```python
from build123d import *

# Parameters (mm, degrees)
SKETCH021_R     = 3.65
SKETCH021_R_2   = 1.6
SKETCH021_W     = 6.5
SKETCH021_H     = 3
SKETCH021_W_2   = 11.5
PAD009_DEPTH    = 9.5
POCKET012_DEPTH = 7
POCKET010_DEPTH = 3.5
SKETCH022_W     = 25.7
SKETCH022_H     = 13
POCKET011_DEPTH = 3
SKETCH023_R     = 1.8
POCKET009_DEPTH = 1.5
FILLET006_R     = 1
FILLET007_R     = 0.99
FILLET008_R     = 0.5


with BuildPart() as part:
    # Sketch021 → Pad009 (new body)
    with BuildSketch(Plane.XY):
        with BuildLine():
            Line((15.5, -31.35), (15.5, -7.25))
            Line((15.5, -7.25), (11, -7.25))
            Line((11, -7.25), (11, 7.25))
            Line((11, 7.25), (15.5, 7.25))
            Line((15.5, 7.25), (15.5, 11.85))
            Line((15.5, 11.85), (-5.5, 11.85))
            ThreePointArc((-5.5, 11.85), (-12.571068, 8.921068), (-15.5, 1.85))
            Line((-15.5, 1.85), (-15.5, -25.57))
            ThreePointArc((-15.5, -25.57), (-14.679899, -27.549899), (-12.7, -28.37))
            Line((-9.7, -28.37), (-12.7, -28.37))
            Line((-9.7, -29.49), (-9.7, -28.37))
            Line((-9.7, -29.49), (7, -29.49))
            Line((7, -29.49), (7, -31.35))
            Line((7, -31.35), (15.5, -31.35))
        make_face()
        Circle(SKETCH021_R, mode=Mode.SUBTRACT)
        with Locations((-11, -12.5)):
            Circle(SKETCH021_R_2, mode=Mode.SUBTRACT)
        with Locations((11, -12.5)):
            Circle(SKETCH021_R_2, mode=Mode.SUBTRACT)
        with Locations((-6, 8.5)):
            Circle(SKETCH021_R_2, mode=Mode.SUBTRACT)
        with Locations((8, 8.5)):
            Circle(SKETCH021_R_2, mode=Mode.SUBTRACT)
        with Locations((-8.91, -25.81)):
            Rectangle(SKETCH021_W, SKETCH021_H, mode=Mode.SUBTRACT)
        with Locations((6.35, -25.81)):
            Rectangle(SKETCH021_W_2, SKETCH021_H, mode=Mode.SUBTRACT)
    extrude(amount=PAD009_DEPTH)

    # Sketch019 (on Face29 of Pad009) → Pocket012 (cut)
    with BuildSketch(Plane.XY.offset(9.5)):
        Polygon((8.25, -4), (6.25, -4), (6.25, -6.25), (-6.25, -6.25), (-6.25, -4), (-8.25, -4), (-8.25, 4), (-6.25, 4), (-6.25, 6.25), (6.25, 6.25), (6.25, 4), (8.25, 4), align=None)
    extrude(amount=-POCKET012_DEPTH, mode=Mode.SUBTRACT)

    # Sketch020 (on Face5 of Pocket012) → Pocket010 (cut)
    with BuildSketch(Plane.XY.offset(9.5)):
        Polygon((-8.1, -14.174316), (-8.1, -10.825684), (-11, -9.151368), (-13.9, -10.825684), (-13.9, -14.174316), (-11, -15.848632), align=None)
        Polygon((13.9, -14.174316), (13.9, -10.825684), (11, -9.151368), (8.1, -10.825684), (8.1, -14.174316), (11, -15.848632), align=None)
    extrude(amount=-POCKET010_DEPTH, mode=Mode.SUBTRACT)

    # Sketch022 (on Face4 of Pocket010) → Pocket011 (cut)
    with BuildSketch(Plane(origin=(0, 0, 0), x_dir=(1, 0, 0), z_dir=(0, 0, -1))):
        with Locations((0, 22)):
            Rectangle(SKETCH022_W, SKETCH022_H)
    extrude(amount=-POCKET011_DEPTH, mode=Mode.SUBTRACT)

    # Sketch023 (on Face7 of Pocket011) → Pocket009 (cut)
    with BuildSketch(Plane(origin=(0, 0, 3), x_dir=(1, 0, 0), z_dir=(0, 0, -1))):
        with Locations((0, 22)):
            Circle(SKETCH023_R)
        with BuildLine():
            Line((1.5, 15.5), (12.85, 15.5))
            Line((12.85, 15.5), (12.85, 20.5))
            Line((12.85, 20.5), (3.5, 20.5))
            ThreePointArc((3.5, 20.5), (2.085786, 19.914214), (1.5, 18.5))
            Line((1.5, 18.5), (1.5, 15.5))
        make_face()
        with BuildLine():
            Line((-1.5, 15.5), (-12.85, 15.5))
            Line((-12.85, 15.5), (-12.85, 20.5))
            Line((-12.85, 20.5), (-3.5, 20.5))
            ThreePointArc((-1.5, 18.5), (-2.085786, 19.914214), (-3.5, 20.5))
            Line((-1.5, 18.5), (-1.5, 15.5))
        make_face()
        with BuildLine():
            Line((12.85, 23.5), (3.5, 23.5))
            ThreePointArc((1.5, 25.5), (2.085786, 24.085786), (3.5, 23.5))
            Line((1.5, 25.5), (1.5, 28.5))
            Line((1.5, 28.5), (12.85, 28.5))
            Line((12.85, 28.5), (12.85, 23.5))
        make_face()
        with BuildLine():
            Line((-12.85, 23.5), (-3.5, 23.5))
            ThreePointArc((-3.5, 23.5), (-2.085786, 24.085786), (-1.5, 25.5))
            Line((-1.5, 25.5), (-1.5, 28.5))
            Line((-1.5, 28.5), (-12.85, 28.5))
            Line((-12.85, 28.5), (-12.85, 23.5))
        make_face()
    extrude(amount=-POCKET009_DEPTH, mode=Mode.SUBTRACT)

    # Fillet006
    fillet006_edges = [part.edges().sort_by_distance(p)[0] for p in [
        (15.5, 11.85, 4.75),
        (15.5, 7.25, 4.75),
        (11, 7.25, 4.75),
        (15.5, -7.25, 4.75),
        (15.5, -31.35, 4.75),
        (7, -31.35, 4.75),
        (-9.7, -29.49, 4.75),
        (11, -7.25, 4.75),
    ]]
    fillet(fillet006_edges, radius=FILLET006_R)

    # Fillet007
    fillet007_edges = [part.edges().sort_by_distance(p)[0] for p in [
        (-8.25, 4, 6),
        (-6.25, 4, 6),
        (-6.25, 6.25, 6),
        (6.25, 4, 6),
        (-6.25, -4, 6),
        (-8.25, -4, 6),
        (-6.25, -6.25, 6),
        (6.25, -6.25, 6),
        (6.25, -4, 6),
        (8.25, -4, 6),
        (6.25, 6.25, 6),
        (8.25, 4, 6),
    ]]
    fillet(fillet007_edges, radius=FILLET007_R)

    # Fillet008
    fillet008_edges = [part.edges().sort_by_distance(p)[0] for p in [
        (-12.85, -15.5, 1.5),
        (-12.85, -15.5, 3.75),
        (-12.16, -24.31, 7),
        (12.85, -15.5, 3.75),
        (12.85, -15.5, 1.5),
        (-1.5, -15.5, 3.75),
        (1.892549, -24.31, 3.75),
        (-5.66, -27.31, 7),
        (-1.5, -28.5, 3.75),
        (-1.8, -22, 4.5),
        (12.1, -27.31, 7),
        (12.85, -28.5, 3.75),
        (12.85, -28.5, 1.5),
        (12.85, -20.5, 3.75),
        (12.85, -23.5, 3.75),
        (1.5, -28.5, 3.75),
        (0.6, -27.31, 6.25),
        (0.6, -24.31, 6.25),
        (1.5, -15.5, 3.75),
        (12.1, -24.31, 7),
        (-5.66, -24.31, 7),
        (-12.85, -23.5, 3.75),
        (-12.85, -20.5, 3.75),
        (7, -29.49, 4.75),
    ]]
    fillet(fillet008_edges, radius=FILLET008_R)


solid = part.part
```
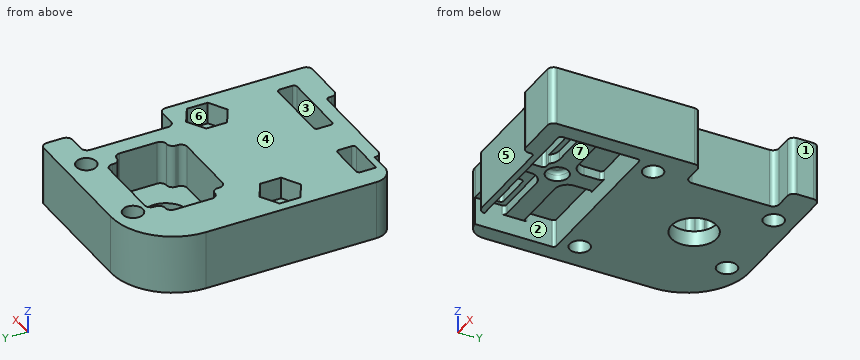
For this review, take the finished solid that the model builds, in its own axes (mm). Face numbers are marked on the shaded views. A direction names the side the tool comes from. Round coordinates to 2 decimals unless told otherwise and drop trailing zeros. Order: outer loops, then holes, each group sorted by start corner. A loop starts at its lowest first (then second) coordinate and runs counter-clockwise, first axis right, second up. Notation, with made-up numbers: (52, 21.25) -> (67, 21.25) arc R13 cw to (67, 26.25) -> close; hole circle Ø3 at (83.25, 62). An arc over 180 degrees is marked (long way). Use a Markdown table: item, result.
Item 1: Take a section at B-B (x = 0). State the section outline as (y, z) points, plus the area to 3 significant figures.
Resolved:
| item | result |
|---|---|
| outline | (-29.49, 0) -> (-28.5, 0) -> (-28.5, 3) -> (-23.8, 3) -> (-23.8, 4) arc R0.5 cw to (-23.3, 4.5) -> (-20.7, 4.5) arc R0.5 cw to (-20.2, 4) -> (-20.2, 3) -> (-15.5, 3) -> (-15.5, 0) -> (-3.65, 0) -> (-3.65, 2.5) -> (-6.25, 2.5) -> (-6.25, 9.5) -> (-29.49, 9.5) -> close; (3.65, 0) -> (11.85, 0) -> (11.85, 9.5) -> (6.25, 9.5) -> (6.25, 2.5) -> (3.65, 2.5) -> close |
| area | 243 mm² |
Item 2: Take a section at D-D (z = 3.5). State how many separate pieces and enclosed holes the cut face has, plus the area to 3 significant figures.
Resolved:
| item | result |
|---|---|
| separate pieces | 1 |
| enclosed holes | 9 |
| area | 747 mm² |
Item 3: Take a section at C-C (y = 1). State the section outline as (x, z) points, plus the area to 3 significant figures.
Resolved:
| item | result |
|---|---|
| outline | (-15.5, 0) -> (-3.51, 0) -> (-3.51, 2.5) -> (-8.25, 2.5) -> (-8.25, 9.5) -> (-15.5, 9.5) -> close; (3.51, 0) -> (11, 0) -> (11, 9.5) -> (8.25, 9.5) -> (8.25, 2.5) -> (3.51, 2.5) -> close |
| area | 119 mm² |
Item 4: Take a section at A-A (y = -12.5). State the section outline as (x, z) points, plus the area to 4 significant figures.
Resolved:
| item | result |
|---|---|
| outline | (-15.5, 0) -> (-12.6, 0) -> (-12.6, 6) -> (-13.9, 6) -> (-13.9, 9.5) -> (-15.5, 9.5) -> close; (-9.4, 0) -> (9.4, 0) -> (9.4, 6) -> (8.1, 6) -> (8.1, 9.5) -> (-8.1, 9.5) -> (-8.1, 6) -> (-9.4, 6) -> close; (12.6, 0) -> (15.5, 0) -> (15.5, 9.5) -> (13.9, 9.5) -> (13.9, 6) -> (12.6, 6) -> close |
| area | 215.5 mm² |
Item 5: Draft analysis for pull direction X (two halves, no side actions). For the marked faces 1, 2, 3 and 4, state which applies: +X half, -X half, draft (parallel to the pull), parting line (faces both ways), or undercut.
Resolved:
| item | result |
|---|---|
| face 1 | +X half |
| face 2 | undercut |
| face 3 | undercut |
| face 4 | draft |
Item 6: For line 1 along Y through (x, z) = (5, 3.5); line 2 along Y through (x, z) = (8, 1.25); line 3 along X through (y, z) = (-22, 3.3), list the stretches that pass through material, from the lowest coordinate up. Write a range as [from, to].
Resolved:
| item | result |
|---|---|
| line 1 | y = [-29.49, -28.5], [-23.5, -20.5], [-15.5, -6.25], [6.25, 11.85] |
| line 2 | y = [-31.35, -28.5], [-15.5, 6.9], [10.1, 11.85] |
| line 3 | x = [-15.5, -1.8], [1.8, 15.5] |
Item 7: For pin 1 (2 mm diameter, centred on x = 2.5, z = 4.5, fed in from -Y); pin 2 (4 mm diameter, centred on y = 0.5, z = 6.5, fed in from +X); pin 3 (3.5 mm diameter, centred on x = -6, y = 8.5, fed in from +Z); pin 4 (3 mm diameter, centred on x = -12, y = -13, fed in from +Z), all flat-tipped, find the tip position at first contact; note any pin that passes through.
Resolved:
| item | result |
|---|---|
| pin 1 | stops at y = -29.49 |
| pin 2 | stops at x = 11 |
| pin 3 | stops at z = 9.5 |
| pin 4 | stops at z = 6 |
Item 8: Machinability: for the marked faces 5, 6 and 7, which of the approach directions +Z, -Z, +X, -X, +Y, -Y give a long, thin tool a straight path to every point of the face, cutting with its end or side? Answer none if there is none.
Resolved:
| item | result |
|---|---|
| face 5 | +Z, -Z, -X, -Y |
| face 6 | +Z |
| face 7 | -Z |
